Read the model definition and answer for the solid it produces. Units are mm, in the model's axes. Face numbers are marked on the shaded views. A direction names the side the tool comes from. Round coordinates to 2 decimals unless told otherwise and drop trailing zeros. Order: outer loops, then holes, each group sorted by start corner. A loop starts at its lowest first (then second) coordinate and runs counter-clockwise, first axis right, second up. Notation, with made-up numbers: M -11.75,9.5 L 11.25,9.5 A35 ccw 11.25,47.5 Z; hole C 20.25,33 d4. An arc over 180 degrees is marked long. Use one line per item in the form item = value. Start each with the question number.
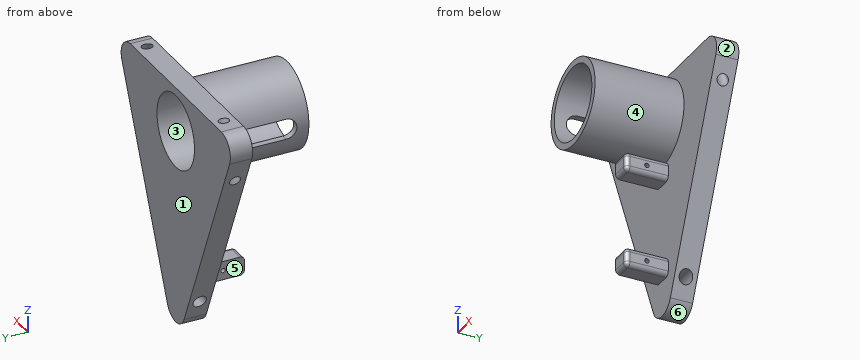
from build123d import *

# Parameters (mm, degrees)
F0_R      = 10.4775
F1_DEPTH  = 6.35
F2_R      = 1.905
F3_DEPTH  = 9.0678
F5_DEPTH  = 12.192
F6_R      = 0.635
F7_R      = 0.635
F8_DEPTH  = 32.5765
F9_R      = 1.27
F10_R     = 12.2682
F10_R_2   = 10.4775
F11_DEPTH = 25.4
F13_DEPTH = 12.7
F14_R     = 1.5875
F16_R     = 1.5875


with BuildPart() as f1:
    # F0 (on Front) → F1 (new body)
    with BuildSketch(Plane.XZ):
        with BuildLine():
            ThreePointArc((-4.6582808724, -27.3922420853), (0, -30.4457132023), (4.6582808724, -27.3922420853))
            Line((4.6582808724, -27.3922420853), (30.0582808724, 30.993471117))
            ThreePointArc((30.0582808724, 30.993471117), (29.6485978114, 35.8049266843), (25.4, 38.1))
            Line((25.4, 38.1), (0, 38.1))
            Line((0, 38.1), (-25.4, 38.1))
            ThreePointArc((-25.4, 38.1), (-29.6485978114, 35.8049266843), (-30.0582808724, 30.993471117))
            Line((-30.0582808724, 30.993471117), (-4.6582808724, -27.3922420853))
        make_face()
        with Locations((0, 25.4)):
            Circle(F0_R, mode=Mode.SUBTRACT)
    extrude(amount=F1_DEPTH)

    # F2 (on Right) → F3 (cut, symmetric)
    with BuildSketch(Plane.YZ):
        with Locations((-3.175, -21.6772420853)):
            Circle(F2_R)
    extrude(amount=F3_DEPTH, both=True, mode=Mode.SUBTRACT)

    # F4 (on face) → F5 (join)
    with BuildSketch(Plane.XZ.offset(6.35)):
        with BuildLine():
            Line((2.2225, 13.0175), (-2.0955, 13.0175))
            Line((-2.0955, 13.0175), (-2.0955, 7.6835))
            Line((-2.0955, 7.6835), (2.2225, 7.6835))
            ThreePointArc((2.2225, 7.6835), (3.1205256121, 8.0554743879), (3.4925, 8.9535))
            Line((3.4925, 8.9535), (3.4925, 11.7475))
            ThreePointArc((3.4925, 11.7475), (3.1205256121, 12.6455256121), (2.2225, 13.0175))
        make_face()
        with BuildLine():
            Line((2.2225, -14.9225), (-2.0955, -14.9225))
            Line((-2.0955, -14.9225), (-2.0955, -20.2565))
            Line((-2.0955, -20.2565), (2.2225, -20.2565))
            ThreePointArc((2.2225, -20.2565), (3.1205256121, -19.8845256121), (3.4925, -18.9865))
            Line((3.4925, -18.9865), (3.4925, -16.1925))
            ThreePointArc((3.4925, -16.1925), (3.1205256121, -15.2944743879), (2.2225, -14.9225))
        make_face()
    extrude(amount=F5_DEPTH)

    # F6 (on face) + F7 (on face) → F8 (cut, through all)
    with BuildSketch(Plane(origin=(-2.0955, 0, 0), x_dir=(0, -1, 0), z_dir=(-1, 0, 0))):
        with Locations((12.446, -17.5895)):
            Circle(F6_R)
    with BuildSketch(Plane(origin=(-2.0955, 0, 0), x_dir=(0, -1, 0), z_dir=(-1, 0, 0))):
        with Locations((12.446, 10.3505)):
            Circle(F7_R)
    extrude(amount=-F8_DEPTH, mode=Mode.SUBTRACT)

    # F9
    f9_edges = [f1.edges().sort_by_distance(p)[0] for p in [
        (0.0635, -18.542, 13.0175),
        (3.120526, -18.542, 12.645526),
        (3.4925, -18.542, 10.3505),
        (3.120526, -18.542, 8.055474),
        (0.0635, -18.542, 7.6835),
        (0.0635, -18.542, -20.2565),
        (3.4925, -18.542, -17.5895),
        (3.120526, -18.542, -15.294474),
        (0.0635, -18.542, -14.9225),
    ]]
    fillet(f9_edges, radius=F9_R)

    # F10 (on face) → F11 (join)
    with BuildSketch(Plane.XZ.offset(6.35)):
        with Locations((0, 25.4)):
            Circle(F10_R)
        with Locations((0, 25.4)):
            Circle(F10_R_2, mode=Mode.SUBTRACT)
    extrude(amount=F11_DEPTH)

    # F12 (on Right) → F13 (cut)
    with BuildSketch(Plane.YZ):
        with BuildLine():
            Line((-25.4, 22.4685867739), (-12.7, 22.4685867739))
            ThreePointArc((-12.7, 22.4685867739), (-9.7685867739, 25.4), (-12.7, 28.3314132261))
            Line((-12.7, 28.3314132261), (-25.4, 28.3314132261))
            ThreePointArc((-25.4, 28.3314132261), (-28.3314132261, 25.4), (-25.4, 22.4685867739))
        make_face()
    extrude(amount=-F13_DEPTH, mode=Mode.SUBTRACT)

    # F15: sweep along a path in F15_path
    with BuildLine(Plane(origin=(30.0582808724, -6.35, 30.993471117), x_dir=(0.3989230085, 0, 0.9169844237), z_dir=(0.9169844237, 0, -0.3989230085))) as f15_path:
        Line((0, 0), (-63.6714339884, 0))
    # F14 (on face) → F15 (sweep, cut)
    with BuildSketch(Plane(origin=(-13.9372156493, 0, -6.0632174906), x_dir=(0, -1, 0), z_dir=(-0.9169844237, 0, -0.3989230085))):
        with Locations((3.175, 32.4612700858)):
            Circle(F14_R)
    sweep(path=f15_path.line, mode=Mode.SUBTRACT)

    # F17: sweep along a path in F17_path
    with BuildLine(Plane(origin=(-4.6582808724, -6.35, -27.3922420853), x_dir=(0.3989230085, 0, -0.9169844237), z_dir=(-0.9169844237, 0, -0.3989230085))) as f17_path:
        Line((0, 0), (-63.6714339884, 0))
    # F16 (on face) → F17 (sweep, cut)
    with BuildSketch(Plane(origin=(13.9372156493, 0, -6.0632174906), x_dir=(0, 1, 0), z_dir=(0.9169844237, 0, -0.3989230085))):
        with Locations((-3.175, 34.4638973475)):
            Circle(F16_R)
    sweep(path=f17_path.line, mode=Mode.SUBTRACT)


solid = f1.part
Item 1: For a pull along Z with two mould halves and no side action, classify the marked faces 1, 2 and 3 as pulls with the +Z half, pulls with the -Z half, needs draft (parallel to the pull), parting line crosses it, or undercut.
Item 2: A tool of negligible diameter and unlimited length cuts with its end or side. For the marked faces 4, 5 and 6, from which of +Z, -Z, +X, -X, +Y, -Y can it reach the whole face along a straight path? Write none if from no direction.
Item 3: Given P1, Ø2, axis at x = 0, y = -13.5, coming from the +Z side; P2, Ø2, axis at x = -13.5, z = -2, coming from the -Y side; P3, Ø3.5, axis at y = -3.18, z = -21.68, coming from the +X side; P4, Ø1.6, axis at y = -10, z = 11, coming from the -X side, each flat-ended and moving along its own axis, determine where each tip first touches the part or whether it passes through.
Item 4: Find the intervals of material crossed by L1, parallel to Z at x = -1.5, y = -8; L2, parallel to Y at x = 26, z = 25; L3, parallel to X at y = -25, z = 29, in increasing order. Write a range as [from, to].
Item 5: Section A-A (x = 0) is taken. Give the number of separate pieces and of enclosed holes in the cut face, and give its area (3 significant figures).
Item 6: Section B-B (z = 18.5) is taken. Write down the section's boundary in (x, y).
Item 7: Section C-C (y = -24.5) is taken. Write down the section's boundary in (x, z) (1 decimal).
Item 8: Section D-D (z = 6) is taken. Write down the section's boundary in (x, y).
The answers:
q1.face_1 = needs draft
q1.face_2 = parting line crosses it
q1.face_3 = undercut
q2.face_4 = -Y
q2.face_5 = -Z, -X, -Y
q2.face_6 = -Z, +Y, -Y
q3.P1 = 37.67
q3.P2 = -6.35
q3.P3 = through
q3.P4 = -2.1
q4.L1 = [-20.26, -14.92], [7.68, 13.02], [13.22, 15.03], [35.77, 37.58]
q4.L2 = [-6.35, 0]
q4.L3 = [-11.73, -9.84], [9.84, 11.73]
q5.separate_pieces = 2
q5.enclosed_holes = 3
q5.area = 508 mm²
q6.outline = M -24.62,-6.35 L -10.14,-6.35 L -10.14,-31.75 L -7.88,-31.75 L -7.88,0 L -24.62,0 Z; M 7.88,-31.75 L 10.14,-31.75 L 10.14,-6.35 L 24.62,-6.35 L 24.62,0 L 7.88,0 Z
q7.outline = M -11.9,22.5 A12.3 ccw long -11.9,28.3 L -10.1,28.3 A10.5 cw long -10.1,22.5 Z
q8.outline = M -19.19,-6.35 L 19.19,-6.35 L 19.19,0 L -19.19,0 Z
